Part model, mm, in its own coordinate system. Face numbers are marked on the shaded views. A direction names the side the tool comes from. Coordinates: 2 decimals unless noted, no trailing zeros. Write each loop counter-clockwise with the first axis right and the second up, starting at its lowest first coordinate (ties: lowest second). Pieces come first, ordered by that corner, then holes. Notation, with made-up numbers: (-19, -7.5) - (24, -7.5) arc R10 ccw to (24, 2.5) - close; hole circle Ø8 at (-33, -31). An arc over 180 degrees is marked (long way). Use a Markdown table: item, result.
```python
from build123d import *

# Parameters (mm, degrees)
BASPROSKE_W          = 3
BASPROSKE_H          = 15
TOOTHCUT_DEPTH       = 22.424285286
TEETHCUTS_COUNT      = 28
TEETHCUTS_ANGLE      = 347.142857143
BORSKE_R             = 4
BORE_DEPTH           = 50.0000508
M3_CLEARANCE_HOLE1_D = 3.4
CIRPATTERN1_COUNT    = 4


with BuildPart() as part:
    # BasProSke → Base-Revolve (revolve)
    with BuildSketch(Plane(origin=(0, 0, 0), x_dir=(1, 0, 0), z_dir=(0, 1, 0)), mode=Mode.PRIVATE) as base_revolve_sk:
        with Locations((1.5, 7.5)):
            Rectangle(BASPROSKE_W, BASPROSKE_H)
    revolve(base_revolve_sk.sketch.rotate(Axis((-10, 0, 0), (1, 0, 0)), 180), axis=Axis((-10, 0, 0), (1, 0, 0)))

    # TooCutSke → ToothCut (cut, through all)
    with BuildSketch(Plane(origin=(0, 0, 0), x_dir=(0, 0, -1), z_dir=(1, 0, 0))):
        with BuildLine():
            ThreePointArc((0.471336039, 12.740284272), (0, 12.749), (-0.471336039, 12.740284272))
            ThreePointArc((-0.471336039, 12.740284272), (-0.81983923, 13.900763331), (-1.409805137, 14.959114099))
            ThreePointArc((-1.409805137, 14.959114099), (0, 15.0254), (1.409805137, 14.959114099))
            ThreePointArc((1.409805137, 14.959114099), (0.81983923, 13.900763331), (0.471336039, 12.740284272))
        make_face()
    toothcut = extrude(amount=TOOTHCUT_DEPTH, mode=Mode.SUBTRACT)

    # TeethCuts: ToothCut ×28 about axis
    teethcuts_axis = Axis((-10, 0, 0), (1, 0, 0))
    for i in range(1, TEETHCUTS_COUNT):
        add(toothcut.rotate(teethcuts_axis, i * TEETHCUTS_ANGLE / (TEETHCUTS_COUNT - 1)), mode=Mode.SUBTRACT)

    # BorSke → Bore (cut, symmetric)
    with BuildSketch(Plane(origin=(0, 0, 0), x_dir=(0, 0, -1), z_dir=(1, 0, 0))):
        with Locations(Location((0, 0, 0), (0, 0, 180))):
            Circle(BORSKE_R)
    extrude(amount=BORE_DEPTH, both=True, mode=Mode.SUBTRACT)

    # M3 Clearance Hole1 (through all)
    with Locations(Plane(origin=(3, 0, 0), x_dir=(0, 0, -1), z_dir=(1, 0, 0))):
        with Locations((0, 7)):
            m3_clearance_hole1 = Hole(M3_CLEARANCE_HOLE1_D / 2)

    # CirPattern1: M3 Clearance Hole1 ×4 about axis
    cirpattern1_axis = Axis((0, 0, 0), (1, 0, 0))
    for i in range(1, CIRPATTERN1_COUNT):
        add(m3_clearance_hole1.rotate(cirpattern1_axis, i * 360 / CIRPATTERN1_COUNT), mode=Mode.SUBTRACT)


solid = part.part
```
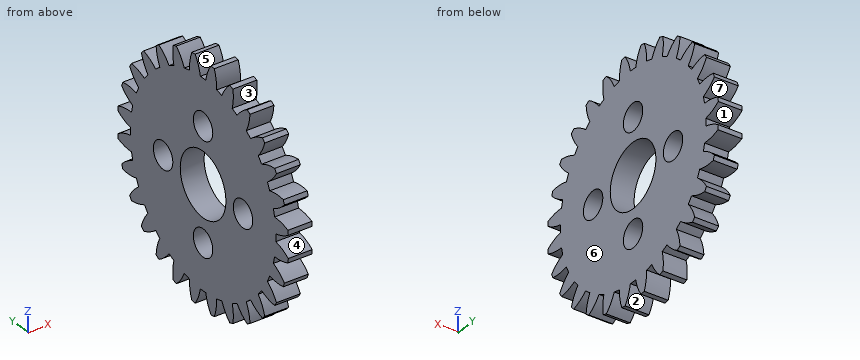
Item 1: Drill centre lines: probe 1 along Y at (x, z) = (2, 0); probe 2 along Z at (x, y) = (0.25, -11.75); probe 3 along Z at (x, y) = (0.6, -0.25). Where is each one in solid material? Low to high.
From the geometry:
| item | result |
|---|---|
| probe 1 | -12.75 to -8.7, -5.3 to -4, 4 to 5.3, 8.7 to 12.75 |
| probe 2 | -8.12 to -6.34, -5.12 to 5.12, 6.34 to 8.12 |
| probe 3 | -12.75 to -8.68, -5.32 to -3.99, 3.99 to 5.32, 8.68 to 12.75 |
Item 2: Drop flat-ended pins along their axis: P1, Ø2.5, axis at y = 7, z = 0, coming from the +X side; P2, Ø1, axis at x = 2.5, z = -5, coming from the -Y side. Give the stop position or say it passes through.
From the geometry:
| item | result |
|---|---|
| P1 | through |
| P2 | y = -14.25 |
Item 3: Two-plate mould, pull along Y, no slides. Class the marked faces 4, 5, 6 and 7: pulls with the +Y half, pulls with the -Y half, needs draft (parallel to the pull), parting line crosses it, or undercut.
From the geometry:
| item | result |
|---|---|
| face 4 | pulls with the -Y half |
| face 5 | undercut |
| face 6 | needs draft |
| face 7 | pulls with the +Y half |
Item 4: Which spindle directions (+Z, -Z, +X, -X, +Y, -Y) get a long thin tool onto all of the face, cutting with end or side? Do the marked faces 1, 2 and 3. Say none if no direction does.
From the geometry:
| item | result |
|---|---|
| face 1 | +X, -X, +Y |
| face 2 | -Z, +X, -X |
| face 3 | +X, -X |
Item 5: Band-saw the part on C-C, the plane x = 0.95. Count the separate pieces of the cut face and the enclosed holes in it, then the cut area to 3 significant figures.
From the geometry:
| item | result |
|---|---|
| separate pieces | 1 |
| enclosed holes | 5 |
| area | 514 mm^2 |
Item 6: Band-saw the part on D-D, the plane y = 7. Give the cut face in (x, z), then the cut area to 3 significant figures.
From the geometry:
| item | result |
|---|---|
| outline | (0, -12.36) - (3, -12.36) - (3, -1.7) - (0, -1.7) - close; (0, 1.7) - (3, 1.7) - (3, 12.36) - (0, 12.36) - close |
| area | 64.0 mm^2 |
Item 7: Band-saw the part on A-A, the plane z = 0. Give the cut face in (x, y).
From the geometry:
| item | result |
|---|---|
| outline | (0, -12.75) - (3, -12.75) - (3, -8.7) - (0, -8.7) - close; (0, -5.3) - (3, -5.3) - (3, -4) - (0, -4) - close; (0, 4) - (3, 4) - (3, 5.3) - (0, 5.3) - close; (0, 8.7) - (3, 8.7) - (3, 12.75) - (0, 12.75) - close |
